CAD build for the part. Positions are in the model's coordinates, mm. Round coordinates to 2 decimals unless told otherwise and drop trailing zeros. Order: outer loops, then holes, each group sorted by start corner. A loop starts at its lowest first (then second) coordinate and runs counter-clockwise, first axis right, second up. Notation, with made-up numbers: (-33, -20) - (12, -20) arc R13 cw to (12, -11) - close; hole circle Ø4 at (58.25, -33.75). An arc over 180 degrees is marked (long way). Write item = value, one per line.
from build123d import *

# Parameters (mm, degrees)
SKETCH1_W           = 76.2
SKETCH1_H           = 50.8
SKETCH1_R           = 20.6375
SKETCH1_R_2         = 2.0828
SKETCH1_R_3         = 1.4224
BOSS_EXTRUDE1_DEPTH = 5.9944


with BuildPart() as part:
    # Sketch1 → Boss-Extrude1 (new body)
    with BuildSketch(Plane.XY):
        Rectangle(SKETCH1_W, SKETCH1_H)
        Circle(SKETCH1_R, mode=Mode.SUBTRACT)
        with Locations((-25.4, 0)):
            Circle(SKETCH1_R_2, mode=Mode.SUBTRACT)
        with Locations((25.4, 0)):
            Circle(SKETCH1_R_2, mode=Mode.SUBTRACT)
        with Locations((-31.75, 19.05)):
            Circle(SKETCH1_R_3, mode=Mode.SUBTRACT)
        with Locations((-31.75, -19.05)):
            Circle(SKETCH1_R_3, mode=Mode.SUBTRACT)
        with Locations((31.75, -19.05)):
            Circle(SKETCH1_R_3, mode=Mode.SUBTRACT)
        with Locations((31.75, 19.05)):
            Circle(SKETCH1_R_3, mode=Mode.SUBTRACT)
    extrude(amount=BOSS_EXTRUDE1_DEPTH)


solid = part.part
(1) Band-saw the part on D-D on x = 0. List the corners of the cut face in (y, z), plus the area to 3 significant figures.
Solved:
outline = (-25.4, 0) - (-20.64, 0) - (-20.64, 5.99) - (-25.4, 5.99) - close; (20.64, 0) - (25.4, 0) - (25.4, 5.99) - (20.64, 5.99) - close
area = 57.1 mm²
(2) Band-saw the part on B-B on y = 0. List the corners of the cut face in (x, z).
Solved:
outline = (-38.1, 0) - (-27.48, 0) - (-27.48, 5.99) - (-38.1, 5.99) - close; (-23.32, 0) - (-20.64, 0) - (-20.64, 5.99) - (-23.32, 5.99) - close; (20.64, 0) - (23.32, 0) - (23.32, 5.99) - (20.64, 5.99) - close; (27.48, 0) - (38.1, 0) - (38.1, 5.99) - (27.48, 5.99) - close
(3) Drop a flat-ended pin along its axis: pin 1 (4.5 mm diameter, centred on x = 31.75, y = 19.05, fed in from -Z). Give the stop position or say it passes through.
Solved:
pin_1 = 0
(4) Pull direction X, two halves, no side cores. Call faces 1 (the flat face through (38.1, 0, 3)), 2 (the flat face through (-17, 12, 5.994)), 3 (the cylindrical face through (32.51, -17.85, 2.96)): released by +X, released by -X, zero draft, split by the parting line, or undercut.
Solved:
face_1 = released by +X
face_2 = zero draft
face_3 = undercut
(5) Band-saw the part on A-A on x = 31.75. List the corners of the cut face in (y, z), plus the area to 3 significant figures.
Solved:
outline = (-25.4, 0) - (-20.47, 0) - (-20.47, 5.99) - (-25.4, 5.99) - close; (-17.63, 0) - (17.63, 0) - (17.63, 5.99) - (-17.63, 5.99) - close; (20.47, 0) - (25.4, 0) - (25.4, 5.99) - (20.47, 5.99) - close
area = 270 mm²
(6) Band-saw the part on C-C on z = 5.2. Count the separate pieces of the cut face and the enclosed holes in it, plus the area to 3 significant figures.
Solved:
separate_pieces = 1
enclosed_holes = 7
area = 2,480 mm²
(7) Probe line 1 along Y through (x, z) = (-31.75, 4.8); line 2 along X through (y, z) = (-2.5, 1.3); line 3 along Y through (x, z) = (-25.4, 4.7). List the from-to ranges inside material, lowest first.
Solved:
line_1 = -25.4 to -20.47, -17.63 to 17.63, 20.47 to 25.4
line_2 = -38.1 to -20.49, 20.49 to 38.1
line_3 = -25.4 to -2.08, 2.08 to 25.4
